from build123d import *

# Parameters (mm, degrees)
SKETCH1_R                    = 5.5
BOSS_EXTRUDE1_DEPTH          = 12
BOSS_EXTRUDE2_DEPTH          = 6
M5_CLEARANCE_HOLE1_D         = 5.5
M5_CLEARANCE_HOLE1_DEPTH     = 12
M5_CLEARANCE_HOLE1_TIP       = 1.652366702
F_3_0_3_DIAMETER_HOLE1_D     = 3
F_3_0_3_DIAMETER_HOLE1_DEPTH = 6
F_3_0_3_DIAMETER_HOLE1_TIP   = 0.901290929
FILLET1_R                    = 0.5


with BuildPart() as part:
    # Sketch1 → Boss-Extrude1 (new body)
    with BuildSketch(Plane(origin=(0, 0, 0), x_dir=(1, 0, 0), z_dir=(0, 1, 0))):
        with Locations(Location((0, 0, 0), (0, 0, 270))):
            Circle(SKETCH1_R)
    extrude(amount=BOSS_EXTRUDE1_DEPTH)

    # Sketch2 → Boss-Extrude2 (add)
    with BuildSketch(Plane(origin=(0, 12, 0), x_dir=(1, 0, 0), z_dir=(0, 1, 0))):
        Polygon((4.42120467, -5.427057146), (6.910571691, 1.115346986), (2.489367021, 6.542404132), (-4.42120467, 5.427057146), (-6.910571691, -1.115346986), (-2.489367021, -6.542404132), align=None)
    extrude(amount=BOSS_EXTRUDE2_DEPTH)

    # M5 Clearance Hole1
    with Locations(Plane.XZ):
        with Locations((0, 0)):
            Hole(M5_CLEARANCE_HOLE1_D / 2, depth=M5_CLEARANCE_HOLE1_DEPTH)
            with Locations((0, 0, -(M5_CLEARANCE_HOLE1_DEPTH + M5_CLEARANCE_HOLE1_TIP / 2))):  # 118° drill point
                Cone(0, M5_CLEARANCE_HOLE1_D / 2, M5_CLEARANCE_HOLE1_TIP, mode=Mode.SUBTRACT)

    # Ø3.0 (3) Diameter Hole1
    with Locations(Plane(origin=(0, 18, 0), x_dir=(1, 0, 0), z_dir=(0, 1, 0))):
        with Locations((0, 0)):
            Hole(F_3_0_3_DIAMETER_HOLE1_D / 2, depth=F_3_0_3_DIAMETER_HOLE1_DEPTH)
            with Locations((0, 0, -(F_3_0_3_DIAMETER_HOLE1_DEPTH + F_3_0_3_DIAMETER_HOLE1_TIP / 2))):  # 118° drill point
                Cone(0, F_3_0_3_DIAMETER_HOLE1_D / 2, F_3_0_3_DIAMETER_HOLE1_TIP, mode=Mode.SUBTRACT)

    # Fillet1
    fillet1_edges = [part.edges().sort_by_distance(p)[0] for p in [
        (-2.489367021, 15, 6.542404132),
        (4.42120467, 15, 5.427057146),
        (6.910571691, 15, -1.115346986),
        (2.489367021, 15, -6.542404132),
        (-4.42120467, 15, -5.427057146),
        (-6.910571691, 15, 1.115346986),
    ]]
    fillet(fillet1_edges, radius=FILLET1_R)


solid = part.part
Work out the finished part from the listing and answer in its coordinate system (mm). A direction names the side the tool comes from. Coordinates: 2 decimals unless noted, no trailing zeros. Write each loop counter-clockwise with the first axis right and the second up, starting at its lowest first coordinate (ties: lowest second). Pieces come first, ordered by that corner, then holes. Notation, with made-up numbers: M 38.25,75 L 77.25,75 A23 ccw 77.25,93 Z; hole C 70,35.5 d3. An arc over 180 degrees is marked long. Use one line per item in the form item = value. Start each with the question number.
1. Each of these flat-tipped pins is pushed along its axis until it touches: P1, Ø4, axis at x = -3, y = 7.5, coming from the +Z side; P2, Ø2, axis at y = 2.5, z = 4.5, coming from the -X side; P3, Ø1, axis at x = 3.5, y = 7.5, coming from the -Z side. Where does it stop, or does it pass through?
2. Straight lines are drawn through the part: probe 1 along X at (y, z) = (11.5, 0); probe 2 along Y at (x, z) = (5, 2.75); probe 3 along Z at (x, y) = (-0.75, 15). For each, find the intervals that lie inside material, in ascending order. Write a range as from..to.
3. The part is cut by section D-D (z = 4.75). Give the vertices of the cut face in (x, y), plus the area to 3 significant figures.
4. The mould has two halves that part along Z. Classify faces 1 (the face through (6, 12, 0)), 2 (the face through (-5.65, 14.96, -2.2)), 3 (the face through (0.596, 6.084, -2.685)), 4 (the face through (1.5, 15.34, -0.07)): released by +Z, released by -Z, zero draft, split by the parting line, or undercut.
5. The part is cut by section C-C (z = 0). Give the vertices of the cut face in (x, y), plus the area to 3 significant figures.
6. The part is cut by section A-A (y = 14). Give the vertices of the cut face in (x, z), plus the area to 3 significant figures.
7. The part is cut by section B-B (x = 0). Give the vertices of the cut face in (y, z), plus the area to 3 significant figures.
8. A tool of negligible diameter and unlimited length cuts with its end or side. For faces 5 (the face through (-5.37, 5.92, -1.19)), 6 (the face through (0, 18, -2)), from which of +Z, -Z, +X, -X, +Y, -Y can it reach the whole face along a straight path? Write none if from no direction.
Evaluation:
q1.P1 = 5.41
q1.P2 = -4.24
q1.P3 = -4.61
q2.probe_1 = -5.5..-2.75, 2.75..5.5
q2.probe_2 = 12..18
q2.probe_3 = -6.02..-1.3, 1.3..6.26
q3.outline = M -3.95,12 L -2.77,12 L -2.77,0 L 2.77,0 L 2.77,12 L 4.68,12 L 4.68,18 L -3.95,18 Z
q3.area = 118 mm^2
q4.face_1 = zero draft
q4.face_2 = released by -Z
q4.face_3 = undercut
q4.face_4 = undercut
q5.outline = M -6.49,12 L -5.5,12 L -5.5,0 L -2.75,0 L -2.75,12 L -1.5,12.75 L -1.5,18 L -6.49,18 Z; M 1.5,12.75 L 2.75,12 L 2.75,0 L 5.5,0 L 5.5,12 L 6.49,12 L 6.49,18 L 1.5,18 Z
q5.area = 125 mm^2
q6.outline = M -6.81,0.85 L -4.52,-5.16 A0.5 ccw -4.14,-5.47 L 2.2,-6.5 A0.5 ccw 2.67,-6.32 L 6.73,-1.34 A0.5 ccw 6.81,-0.85 L 4.52,5.16 A0.5 ccw 4.14,5.47 L -2.2,6.5 A0.5 ccw -2.67,6.32 L -6.73,1.34 A0.5 ccw Z; hole C 0,0 d3
q6.area = 120 mm^2
q7.outline = M 0,-5.5 L 12,-5.5 L 12,-6.14 L 18,-6.14 L 18,-1.5 L 12.75,-1.5 L 12,-2.75 L 0,-2.75 Z; M 0,2.75 L 12,2.75 L 12.75,1.5 L 18,1.5 L 18,6.14 L 12,6.14 L 12,5.5 L 0,5.5 Z
q7.area = 121 mm^2
q8.face_5 = -Y
q8.face_6 = +Z, -Z, +X, -X, +Y
